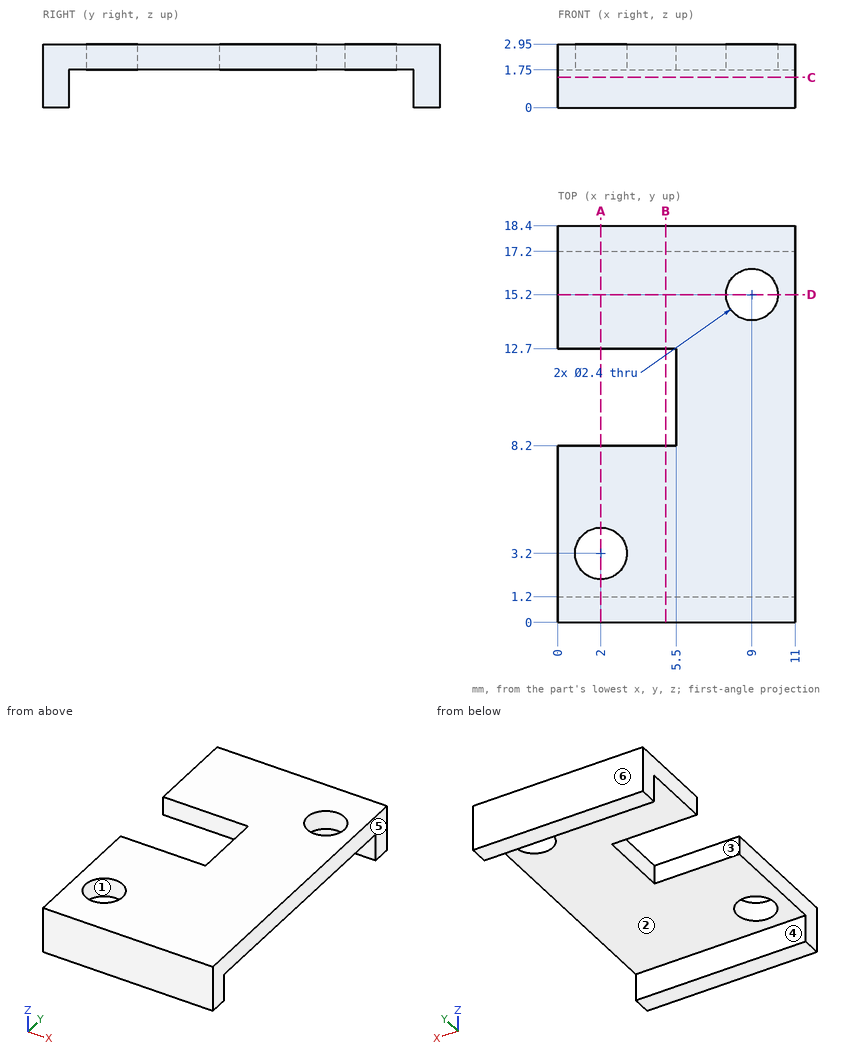
Source: three-view drawing plus pictorial views. Frame: mm from the lowest corner of the part. A direction names the side the tool comes from. Round coordinates to 2 decimals unless told otherwise and drop trailing zeros. Loops run counter-clockwise (first coordinate to the right, second up) from the corner with the lowest first, then second, coordinate; pieces in that order, holes last.
Q1. Section A-A, the plane x = 2. Return loops of the section in (y, z).
Q2. First-contact query: P1, Ø3.5, axis at x = 3, y = 7, coming from the -Z side; P2, Ø0.6, axis at y = 10, z = 2.5, coming from the -X side. Flat tips, straight axial feed; report the tip coordinate or a pass-through.
Q3. Mould query, pull axis Y, two halves, no side actions, for the marked faces 4, 5 and 6. Classes: pulls with the +Y half, pulls with the -Y half, needs draft (parallel to the pull), parting line crosses it, or undercut.
Q4. Section C-C, the plane z = 1.4. Return loops of the section in (x, y), plus the area to 3 significant figures.
Q5. Section B-B, the plane x = 5. Return loops of the section in (y, z).
Q6. Ray query, line 1 (X direction, y = 15.2, z = 2.55); line 2 (X direction, y = 3.2, z = 2.35); line 3 (Y direction, x = 4, z = 1.6). Return the intervals inside material, ascending.
Q7. Access query for the marked faces 1, 2 and 3. Directions: +Z, -Z, +X, -X, +Y, -Y. A direction counts if a zero-diameter tool reaches every point of the face in a straight line with its end or side. Return the directions, or none.
Q8. Section D-D, the plane y = 15.2. Return loops of the section in (x, z), plus the area to 3 significant figures.
Solutions:
1. outline: (0, 0) - (1.2, 0) - (1.2, 1.75) - (2, 1.75) - (2, 2.95) - (0, 2.95) - close; (4.4, 1.75) - (8.2, 1.75) - (8.2, 2.95) - (4.4, 2.95) - close; (12.7, 1.75) - (17.2, 1.75) - (17.2, 0) - (18.4, 0) - (18.4, 2.95) - (12.7, 2.95) - close
2. P1: stops at z = 1.75
2. P2: stops at x = 5.5
3. face 4: undercut
3. face 5: needs draft
3. face 6: pulls with the +Y half
4. outline: (0, 0) - (11, 0) - (11, 1.2) - (0, 1.2) - close; (0, 17.2) - (11, 17.2) - (11, 18.4) - (0, 18.4) - close
4. area: 26.4 mm2
5. outline: (0, 0) - (1.2, 0) - (1.2, 1.75) - (8.2, 1.75) - (8.2, 2.95) - (0, 2.95) - close; (12.7, 1.75) - (17.2, 1.75) - (17.2, 0) - (18.4, 0) - (18.4, 2.95) - (12.7, 2.95) - close
6. line 1: x = 0 to 7.8, 10.2 to 11
6. line 2: x = 0 to 0.8, 3.2 to 11
6. line 3: y = 0 to 1.2, 17.2 to 18.4
7. face 1: +Z, -Z
7. face 2: -Z, +X, -X
7. face 3: +Z, -Z, -X
8. outline: (0, 1.75) - (7.8, 1.75) - (7.8, 2.95) - (0, 2.95) - close; (10.2, 1.75) - (11, 1.75) - (11, 2.95) - (10.2, 2.95) - close
8. area: 10.3 mm2
